Could you check a few things on this model? Use its own coordinates, in mm. Give positions to 0.01 mm unless a question says otherwise; leave off trailing zeros. Order: outer loops, then holes, each group sorted by start corner. A loop starts at its lowest first (then second) coordinate and runs counter-clockwise, first axis right, second up. Notation, with made-up numbers: (10.25, -8.5) -> (36.25, -8.5) arc R27 cw to (36.25, 27.5) -> close; hole circle Ø5 at (68, 87.25). An arc over 180 degrees is marked (long way). Use one line per item in the form item = value. Start each with the question number.
from build123d import *

# Parameters (mm, degrees)
F1_DEPTH = 67.6
F2_R     = 25
F3_DEPTH = 67.6


with BuildPart() as f1:
    # F0 (on Front) → F1 (new body)
    with BuildSketch(Plane.XZ):
        with BuildLine():
            Line((40, -110), (40, 110))
            ThreePointArc((40, 110), (28.284271, 138.284271), (0, 150))
            ThreePointArc((0, 150), (-28.284271, 138.284271), (-40, 110))
            Line((-40, 110), (-40, -110))
            ThreePointArc((-40, -110), (-28.284271, -138.284271), (0, -150))
            ThreePointArc((0, -150), (28.284271, -138.284271), (40, -110))
        make_face()
    extrude(amount=F1_DEPTH)

    # F2 (on face) → F3 (cut, through all)
    with BuildSketch(Plane.XZ.offset(67.6)):
        with Locations((0, 110)):
            Circle(F2_R)
        with Locations((0, -110)):
            Circle(F2_R)
    extrude(amount=-F3_DEPTH, mode=Mode.SUBTRACT)


solid = f1.part
(1) Imagine slicing it at C-C (x = -9). Write out the boundary of the cut face in (y, z).
(2) I'm going to push flat-ended pins straight in: pin 1 Ø12 at (x, z) = (20.5, 79) entering from +Y; pin 2 Ø1 at (x, y) = (29, -19.5) entering from +Z; pin 3 Ø2 at (x, y) = (2.5, -19) entering from -Z; pin 4 Ø4 at (x, y) = (-5, -60.5) entering from -Z. Where does each tip first touch, or does it pass through?
(3) Imagine slicing it at A-A (y = -28.5). Write out the boundary of the cut face in (x, z).
(4) We'd pull the mould along X, two halves only. Please class faces 1 (the cylindrical face through (-3.255, -34.273, 134.787)), 2 (the flat face through (-40, -33, 2)), 3 (the flat face through (-1, 0, 2)): pulls with the +X half, pulls with the -X half, needs draft (parallel to the pull), parting line crosses it, or undercut.
(5) Imagine slicing it at B-B (z = 103.5). Write out the boundary of the cut face in (x, y).
(6) Imagine slicing it at D-D (x = 30.5). Write out the boundary of the cut face in (y, z), plus the area to 3 significant figures.
(7) Please list where these lines run through material, in increasing order: probe 1 along Z at (x, y) = (22, -45); probe 2 along Z at (x, y) = (-12, -9.5); probe 3 along X at (y, z) = (-54, -120).
Calculated:
q1.outline = (-67.6, -148.97) -> (0, -148.97) -> (0, -133.32) -> (-67.6, -133.32) -> close; (-67.6, -86.68) -> (0, -86.68) -> (0, 86.68) -> (-67.6, 86.68) -> close; (-67.6, 133.32) -> (0, 133.32) -> (0, 148.97) -> (-67.6, 148.97) -> close
q2.pin_1 = 0
q2.pin_2 = 138.07
q2.pin_3 = -149.97
q2.pin_4 = -149.89
q3.outline = (-40, -110) arc R40 ccw to (0, -150) arc R40 ccw to (40, -110) -> (40, 110) arc R40 ccw to (0, 150) arc R40 ccw to (-40, 110) -> close; hole circle Ø50 at (0, -110); hole circle Ø50 at (0, 110)
q4.face_1 = undercut
q4.face_2 = pulls with the -X half
q4.face_3 = needs draft
q5.outline = (-40, -67.6) -> (-24.14, -67.6) -> (-24.14, 0) -> (-40, 0) -> close; (24.14, -67.6) -> (40, -67.6) -> (40, 0) -> (24.14, 0) -> close
q6.outline = (-67.6, -135.88) -> (0, -135.88) -> (0, 135.88) -> (-67.6, 135.88) -> close
q6.area = 18,400 mm2
q7.probe_1 = -143.41 to -121.87, -98.13 to 98.13, 121.87 to 143.41
q7.probe_2 = -148.16 to -131.93, -88.07 to 88.07, 131.93 to 148.16
q7.probe_3 = -38.73 to -22.91, 22.91 to 38.73
